Source: CAD feature listing. Evaluate the final solid. Frame: model axes, mm. A direction names the side the tool comes from. Coordinates: 2 decimals unless noted, no trailing zeros. Loops run counter-clockwise (first coordinate to the right, second up) from the corner with the lowest first, then second, coordinate; pieces in that order, holes last. Notation, with made-up numbers: (28.25, 19) - (69.25, 19) arc R13 cw to (69.25, 38) - close; hole circle Ø10 at (8.5, 53.5). An arc over 180 degrees is marked (long way). Write item = value, one per line. Start each with the question number.
from build123d import *

# Parameters (mm, degrees)
F1_DEPTH = 100
F3_DEPTH = 2
F4_W     = 2
F4_H     = 298.6636427242
F5_DEPTH = 2
F7_DEPTH = 1


with BuildPart() as f1:
    # F0 (on Right) → F1 (new body, symmetric)
    with BuildSketch(Plane.YZ):
        Polygon((-300, 0), (0, 0), (65.0561835021, 157.0595205269), (178.0561835021, 157.0595205269), (178.0561835021, 159.0595205269), (63.7198262262, 159.0595205269), (63.2071728736, 157.8218658503), (-1.3363572758, 2), (-300, 2), align=None)
    extrude(amount=F1_DEPTH, both=True)

    # F2 (on face) → F3 (cut)
    with BuildSketch(Plane.XY.offset(2)):
        Polygon((-50, -1.3363572758), (-100, -1.3363572758), (-100, -300), (-1, -300), align=None)
        Polygon((100, -300), (100, -1.3363572758), (50, -1.3363572758), (1, -300), align=None)
    extrude(amount=-F3_DEPTH, mode=Mode.SUBTRACT)

    # F4 (on face) → F5 (cut)
    with BuildSketch(Plane.XY.offset(2)):
        with Locations((0, -150.6681786379)):
            Rectangle(F4_W, F4_H)
    extrude(amount=-F5_DEPTH, mode=Mode.SUBTRACT)

    # F6 (on Right) → F7 (join, symmetric)
    with BuildSketch(Plane.YZ):
        with BuildLine():
            Line((0, -25), (0, 0))
            Line((0, 0), (-1.3218912033, 0))
            Line((-1.3218912033, 0), (-1.3218912033, 1.994008737))
            Line((-1.3218912033, 1.994008737), (63.7198262262, 159.0595205269))
            Line((63.7198262262, 159.0595205269), (123.7198262262, 159.0595205269))
            Line((123.7198262262, 159.0595205269), (123.7198262262, 169.0595205269))
            ThreePointArc((123.7198262262, 169.0595205269), (120.7908940381, 176.1305883388), (113.7198262262, 179.0595205269))
            Line((113.7198262262, 179.0595205269), (25.1346510755, 179.0595205269))
            ThreePointArc((25.1346510755, 179.0595205269), (19.5789487453, 177.3742166499), (15.8958557504, 172.8863548506))
            Line((15.8958557504, 172.8863548506), (-22.0929910541, 81.1731656763))
            ThreePointArc((-22.0929910541, 81.1731656763), (-25.776084049, 76.685303877), (-31.3317863792, 75))
            Line((-31.3317863792, 75), (-374.65, 75))
            Line((-374.65, 75), (-374.65, -25))
            Line((-374.65, -25), (0, -25))
        make_face()
    extrude(amount=F7_DEPTH, both=True)


solid = f1.part
Item 1: Cut plane D-D (x = 27). Return the cut outline in (y, z).
Item 2: Cut plane B-B (x = -82). Return the cut outline in (y, z).
Item 3: Cut plane C-C (y = -264.5). Return the cut outline in (x, z).
Item 4: Material intervals for L1, parallel to Z at x = -2.5, y = -30; L2, parallel to X at y = -264.5, z = 74; L3, parallel to Z at x = -83, y = 78, sorted ascending. Write a range as [from, to].
Item 5: Cut plane A-A (y = 99). Return the cut outline in (x, z), then the cut area to 3 significant figures.
Item 6: Reachability of faces 1 (the flat face through (1, 121, 157.06)), 2 (the flat face through (-1, -129, 33)), 3 (the flat face through (-21, -106, 0)), 4 (the flat face through (15, -82, 2)) from +Z, -Z, +X, -X, +Y, -Y: full face, straight path, thin tool, end or side. Return the list, or none.
Item 7: First-contact query: pin 1 (0.6 mm diameter, centred on x = 0, z = -7.5, fed in from +Y); pin 2 (0.6 mm diameter, centred on x = 0, z = 162, fed in from +Y); pin 3 (12 mm diameter, centred on x = 4.5, z = 44, fed in from +Y). Flat tips, straight axial feed; report the tip coordinate or a pass-through.
Responses:
q1.outline = (-141.53, 0) - (0, 0) - (65.06, 157.06) - (178.06, 157.06) - (178.06, 159.06) - (63.72, 159.06) - (-1.34, 2) - (-141.53, 2) - close
q2.outline = (-1.34, 0) - (0, 0) - (65.06, 157.06) - (178.06, 157.06) - (178.06, 159.06) - (63.72, 159.06) - (-1.34, 2) - close
q3.outline = (-6.82, 0) - (-1, 0) - (-1, -25) - (1, -25) - (1, 0) - (6.82, 0) - (6.82, 2) - (1, 2) - (1, 75) - (-1, 75) - (-1, 2) - (-6.82, 2) - close
q4.L1 = [0, 2]
q4.L2 = [-1, 1]
q4.L3 = [157.06, 159.06]
q5.outline = (-100, 157.06) - (100, 157.06) - (100, 159.06) - (1, 159.06) - (1, 179.06) - (-1, 179.06) - (-1, 159.06) - (-100, 159.06) - close
q5.area = 440 mm2
q6.face_1 = -Z, +X, -X, +Y
q6.face_2 = -X, -Y
q6.face_3 = -Z, -X, +Y, -Y
q6.face_4 = +Z, +X, -Y
q7.pin_1 = 0
q7.pin_2 = 123.72
q7.pin_3 = 20.71
